The model under review builds one solid part; all positions refer to its coordinate system, in mm. Face numbers are marked on the shaded views. A direction names the side the tool comes from. Coordinates: 2 decimals unless noted, no trailing zeros. Order: outer loops, then holes, each group sorted by start corner. A loop starts at its lowest first (then second) coordinate and runs counter-clockwise, first axis right, second up. Notation, with made-up numbers: M -5,15.25 L 35,15.25 A21 ccw 35,48.25 Z; hole C 40,-12.75 d6. An arc over 180 degrees is marked long. One line per item, written item: value.
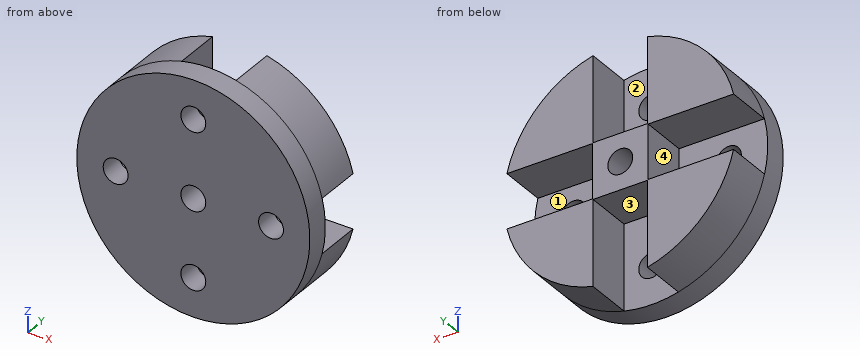
```python
from build123d import *

# Parameters (mm, degrees)
SKETCH1_R           = 15
SKETCH1_R_2         = 1.6
BOSS_EXTRUDE1_DEPTH = 3
SKETCH2_R           = 1.6
BOSS_EXTRUDE2_DEPTH = 6


with BuildPart() as part:
    # Sketch1 → Boss-Extrude1 (new body)
    with BuildSketch(Plane(origin=(0, 0, 0), x_dir=(1, 0, 0), z_dir=(0, 1, 0))):
        with Locations(Location((0, 0, 0), (0, 0, 270))):
            Circle(SKETCH1_R)
        with Locations(Location((0, 0, 0), (0, 0, 270))):
            Circle(SKETCH1_R_2, mode=Mode.SUBTRACT)
        with Locations(Location((0, 10, 0), (0, 0, 270))):
            Circle(SKETCH1_R_2, mode=Mode.SUBTRACT)
        with Locations(Location((10, 0, 0), (0, 0, 270))):
            Circle(SKETCH1_R_2, mode=Mode.SUBTRACT)
        with Locations(Location((0, -10, 0), (0, 0, 270))):
            Circle(SKETCH1_R_2, mode=Mode.SUBTRACT)
        with Locations(Location((-10, 0, 0), (0, 0, 270))):
            Circle(SKETCH1_R_2, mode=Mode.SUBTRACT)
    extrude(amount=BOSS_EXTRUDE1_DEPTH)

    # Sketch2 → Boss-Extrude2 (add)
    with BuildSketch(Plane(origin=(0, 3, 0), x_dir=(1, 0, 0), z_dir=(0, 1, 0))):
        with BuildLine():
            Line((-3.585952146, -3.5), (-14.585952146, -3.5))
            ThreePointArc((-14.585952146, -3.5), (-10.606601718, -10.606601718), (-3.5, -14.585952146))
            Line((-3.5, -14.585952146), (-3.5, -3.585952146))
            Line((-3.5, -3.585952146), (3.5, -3.585952146))
            Line((3.5, -3.585952146), (3.5, -14.585952146))
            ThreePointArc((3.5, -14.585952146), (10.606601718, -10.606601718), (14.585952146, -3.5))
            Line((14.585952146, -3.5), (3.585952146, -3.5))
            Line((3.585952146, -3.5), (3.585952146, 3.5))
            Line((3.585952146, 3.5), (14.585952146, 3.5))
            ThreePointArc((14.585952146, 3.5), (10.606601718, 10.606601718), (3.5, 14.585952146))
            Line((3.5, 14.585952146), (3.5, 3.585952146))
            Line((3.5, 3.585952146), (-3.5, 3.585952146))
            Line((-3.5, 3.585952146), (-3.5, 14.585952146))
            ThreePointArc((-3.5, 14.585952146), (-10.606601718, 10.606601718), (-14.585952146, 3.5))
            Line((-14.585952146, 3.5), (-3.585952146, 3.5))
            Line((-3.585952146, 3.5), (-3.585952146, -3.5))
        make_face()
        with Locations(Location((0, 0, 0), (0, 0, 270))):
            Circle(SKETCH2_R, mode=Mode.SUBTRACT)
    extrude(amount=BOSS_EXTRUDE2_DEPTH)


solid = part.part
```
(1) We need section C-C, the plane x = 0. State the section outline as (y, z) points, plus the area to 3 significant figures.
Geometry results:
outline: M 0,-15 L 3,-15 L 3,-11.6 L 0,-11.6 Z; M 0,-8.4 L 3,-8.4 L 3,-3.59 L 9,-3.59 L 9,-1.6 L 0,-1.6 Z; M 0,1.6 L 9,1.6 L 9,3.59 L 3,3.59 L 3,8.4 L 0,8.4 Z; M 0,11.6 L 3,11.6 L 3,15 L 0,15 Z
area: 85.0 mm2
(2) Insertion check: pin 1 Ø1 at (y, z) = (7, 11) entering from -X; pin 2 Ø5 at (y, z) = (7, 11.5) entering from +X; pin 3 Ø3 at (y, z) = (6, 8.5) entering from -X. Each pin has a flat end and moves straight along its axis. Give the tip position at first contact, or say it passes through.
Geometry results:
pin 1: stops at x = -10.71
pin 2: stops at x = 12
pin 3: stops at x = -13.27
(3) Tool access review of the marked faces 1, 2, 3 and 4: name each direction out of +Z, -Z, +X, -X, +Y, -Y from which nothing blocks a thin tool from reaching the whole face with its end or side.
Geometry results:
face 1: +X, +Y
face 2: +Z, +Y
face 3: -Z, +Y
face 4: -X, +Y
(4) We need section A-A, the plane z = 0. State the section outline as (x, y) points, plus the area to 3 significant figures.
Geometry results:
outline: M -15,0 L -11.6,0 L -11.6,3 L -15,3 Z; M -8.4,0 L -1.6,0 L -1.6,9 L -3.59,9 L -3.59,3 L -8.4,3 Z; M 1.6,0 L 8.4,0 L 8.4,3 L 3.59,3 L 3.59,9 L 1.6,9 Z; M 11.6,0 L 15,0 L 15,3 L 11.6,3 Z
area: 85.0 mm2
(5) We need section D-D, the plane z = 8.75. State the section outline as (x, y) points, plus the area to 3 significant figures.
Geometry results:
outline: M -12.18,0 L -1,0 L -1,3 L -3.5,3 L -3.5,9 L -12.18,9 Z; M 1,0 L 12.18,0 L 12.18,9 L 3.5,9 L 3.5,3 L 1,3 Z
area: 171 mm2
(6) For L1, parallel to X at y = 0.7, z = 0; L2, parallel to X at y = 4, z = 0; L3, parallel to X at y = 5.75, z = -10.75, list the stretches that pass through material, from the lowest coordinate up.
Geometry results:
L1: x = -15 to -11.6, -8.4 to -1.6, 1.6 to 8.4, 11.6 to 15
L2: x = -3.59 to -1.6, 1.6 to 3.59
L3: x = -10.46 to -3.5, 3.5 to 10.46
(7) We need section B-B, the plane y = 7.5. State the section outline as (x, z) points, plus the area to 3 significant figures.
Geometry results:
outline: M -14.59,-3.5 A15 ccw -3.5,-14.59 L -3.5,-3.59 L 3.5,-3.59 L 3.5,-14.59 A15 ccw 14.59,-3.5 L 3.59,-3.5 L 3.59,3.5 L 14.59,3.5 A15 ccw 3.5,14.59 L 3.5,3.59 L -3.5,3.59 L -3.5,14.59 A15 ccw -14.59,3.5 L -3.59,3.5 L -3.59,-3.5 Z; hole C 0,0 d3.2
area: 383 mm2
